```python
from build123d import *

# Parameters (mm, degrees)
BOSS_EXTRUDE2_DEPTH = 10
BOSS_EXTRUDE3_DEPTH = 30
CUT_EXTRUDE1_DEPTH  = 5


with BuildPart() as part:
    # Sketch1 → Boss-Extrude2 (new body)
    with BuildSketch(Plane.XY):
        with BuildLine():
            Line((-2.416609195, 3.25), (2.416609195, 3.25))
            ThreePointArc((2.416609195, 3.25), (4.05, 0), (2.416609195, -3.25))
            Line((2.416609195, -3.25), (-2.416609195, -3.25))
            ThreePointArc((-2.416609195, -3.25), (-4.05, 0), (-2.416609195, 3.25))
        make_face()
    extrude(amount=BOSS_EXTRUDE2_DEPTH)

    # Sketch4 → Boss-Extrude3 (add)
    with BuildSketch(Plane.XY.offset(10)):
        Polygon((1.730250139, -3.001038896), (3.464100991, -0.002078873), (1.733850853, 2.998960023), (-1.730250139, 3.001038896), (-3.464100991, 0.002078873), (-1.733850853, -2.998960023), align=None)
    extrude(amount=BOSS_EXTRUDE3_DEPTH)

    # Sketch3 → Cut-Extrude1 (cut)
    with BuildSketch(Plane(origin=(0, 0, 0), x_dir=(-1, 0, 0), z_dir=(0, 0, -1))):
        with BuildLine():
            Line((2.19089023, 2.6), (-2.19089023, 2.6))
            ThreePointArc((-2.19089023, 2.6), (-3.4, 0), (-2.19089023, -2.6))
            Line((-2.19089023, -2.6), (2.19089023, -2.6))
            ThreePointArc((2.19089023, -2.6), (3.4, 0), (2.19089023, 2.6))
        make_face()
    extrude(amount=-CUT_EXTRUDE1_DEPTH, mode=Mode.SUBTRACT)


solid = part.part
```
The listing builds one solid part. Answer for the finished solid, in the listing's coordinates (mm). A direction names the side the tool comes from. Round coordinates to 2 decimals unless told otherwise and drop trailing zeros. Loops run counter-clockwise (first coordinate to the right, second up) from the corner with the lowest first, then second, coordinate; pieces in that order, holes last.
Q1. For a pull along Y with two mould halves and no side action, classify faces 1 (the face through (2.6, -1.5, 24.8)), 2 (the face through (0, 2.6, 2)), 3 (the face through (2.6, 1.5, 24.8)) as released by +Y, released by -Y, zero draft, split by the parting line, or undercut.
Q2. Section B-B, the plane z = 30 is taken. Determine the outline of the cut face in (x, y), then the cut area to 3 significant figures.
Q3. Section D-D, the plane y = 0.75 is taken. Determine the outline of the cut face in (x, z), then the cut area to 3 significant figures.
Q4. Given pin 1 Ø1.5 at (x, z) = (-1.5, 35) entering from +Y, flat-ended and moving along its own axis, determine where the tip first touches the part or whether it passes through.
Q5. Section A-A, the plane z = 4.5 is taken. Determine the outline of the cut face in (x, y).
Q6. Section C-C, the plane x = 2.75 is taken. Determine the outline of the cut face in (y, z), then the cut area to 3 significant figures.
Q7. Which of the six approach directions +Z, -Z, +X, -X, +Y, -Y give full straight-line access (tool end or side, diameter ignored) to faces 4 (the face through (3.4, 0, 2.5)), 5 (the face through (-2.6, -1.5, 24.8)), 6 (the face through (3, 2, 10))?
Q8. Find the intervals of material crossed by line 1 (Z direction, x = -1, y = -1.75); line 2 (Y direction, x = 0, z = 33); line 3 (X direction, y = -1.75, z = 2.5), in increasing order.
Completed:
1. face 1: released by -Y
1. face 2: undercut
1. face 3: released by +Y
2. outline: (-3.46, 0) - (-1.73, -3) - (1.73, -3) - (3.46, 0) - (1.73, 3) - (-1.73, 3) - close
2. area: 31.2 mm2
3. outline: (-3.98, 0) - (-3.32, 0) - (-3.32, 5) - (3.32, 5) - (3.32, 0) - (3.98, 0) - (3.98, 10) - (3.03, 10) - (3.03, 40) - (-3.03, 40) - (-3.03, 10) - (-3.98, 10) - close
3. area: 228 mm2
4. pin 1: stops at y = 3
5. outline: (-2.42, -3.25) - (2.42, -3.25) arc R4.05 ccw to (2.42, 3.25) - (-2.42, 3.25) arc R4.05 ccw to start; hole (-2.19, -2.6) - (2.19, -2.6) arc R3.4 ccw to (2.19, 2.6) - (-2.19, 2.6) arc R3.4 ccw to start
6. outline: (-2.97, 0) - (-2, 0) - (-2, 5) - (2, 5) - (2, 0) - (2.97, 0) - (2.97, 10) - (1.24, 10) - (1.24, 40) - (-1.24, 40) - (-1.24, 10) - (-2.97, 10) - close
6. area: 114 mm2
7. face 4: -Z
7. face 5: +Z, -X, -Y
7. face 6: +Z
8. line 1: z = 5 to 40
8. line 2: y = -3 to 3
8. line 3: x = -3.65 to -2.92, 2.92 to 3.65
